Read the model definition and answer for the solid it produces. Units are mm, in the model's axes. Face numbers are marked on the shaded views. A direction names the side the tool comes from. Coordinates: 2 decimals unless noted, no trailing zeros. Loops run counter-clockwise (first coordinate to the right, second up) from the corner with the lowest first, then second, coordinate; pieces in that order, holes last. Notation, with made-up numbers: (-27.5, 36) -> (-8.5, 36) arc R26 ccw to (-8.5, 52) -> close; hole circle Ø4 at (6.25, -36). An arc over 180 degrees is marked (long way). Answer as a JSON object with one key per item and string values. Group by question number.
Q1. Straight lines are drawn through the part: line 1 along Y through (x, z) = (3.35, 68); line 2 along Y through (x, z) = (3.95, 68.5); line 3 along Z through (x, y) = (3.9, -13.5). For each, find the intervals that lie inside material, in ascending order. Write a range as [from, to].
Q2. The part is cut by section B-B on z = 68. Write down the section's boundary in (x, y) (3 decimals).
Q3. The part is cut by section A-A on y = 14.5. Write down the section's boundary in (x, z), and give its area (3 significant figures).
Q4. Determine the mould class of the marked faces 1, 2 and 3 for opening direction X: released by +X, released by -X, zero draft, split by the parting line, or undercut.
Q5. The part is cut by section D-D on x = 7.8. Write down the section's boundary in (y, z) (3 decimals).
Q6. For the marked faces 4, 5 and 6, determine the directions among +Z, -Z, +X, -X, +Y, -Y from which every point of the face is accessible in a straight line to the end or side of a thin tool.
Q7. Each of these flat-tipped pins is pushed along its axis until it touches: P1, Ø2.5, axis at x = 6.5, z = 68, coming from the +Y side (3 decimals); P2, Ø2.5, axis at y = 13.5, z = 68.5, coming from the +X side; P3, Ø4, axis at y = 14.5, z = 68, coming from the -X side; P4, Ø4, axis at y = -13.5, z = 69, coming from the +X side. Where does it stop, or does it pass through?
Q8. The part is cut by section C-C on x = 3.2. Write down the section's boundary in (y, z).
from build123d import *

# Parameters (mm, degrees)
PAD010_DEPTH            = 8
SKETCH006_R             = 1.5
POCKET013_DEPTH         = 5
FILLET007_R             = 2
BODY002_PITCH_ANGLE     = -90
BODY002_PLACEMENT_ANGLE = -180


with BuildPart() as part:
    # Sketch005 → Pad010 (new body)
    with BuildSketch(Plane.YZ):
        Polygon((-17, -5), (-11.875, -5), (-11.875, -1.6), (10.875, -1.6), (10.875, -5), (16, -5), (16, -7), (-17, -7), align=None)
    extrude(amount=PAD010_DEPTH)

    # Sketch006 (on Face7 of Pad010) → Pocket013 (cut)
    with BuildSketch(Plane.YX.offset(7)):
        with Locations((-14.5, 4)):
            Circle(SKETCH006_R)
        with Locations((13.5, 4)):
            Circle(SKETCH006_R)
    extrude(amount=-POCKET013_DEPTH, mode=Mode.SUBTRACT)

    # Fillet007
    fillet007_edges = [part.edges().sort_by_distance(p)[0] for p in [
        (8, -17, -6),
        (0, -17, -6),
        (8, 16, -6),
        (0, 16, -6),
    ]]
    fillet(fillet007_edges, radius=FILLET007_R)


with BuildPart() as part_1:
    # Body002 pitch: moved
    add(part.part.rotate(Axis((0, 0, 0), (0, 1, 0)), BODY002_PITCH_ANGLE))


with BuildPart() as part_2:
    # Body002 placement: moved
    add(part_1.part.moved(Location((9.75, 0, 64))).rotate(Axis((9.75, 0, 64), (0, 0, 1)), BODY002_PLACEMENT_ANGLE))


solid = part_2.part
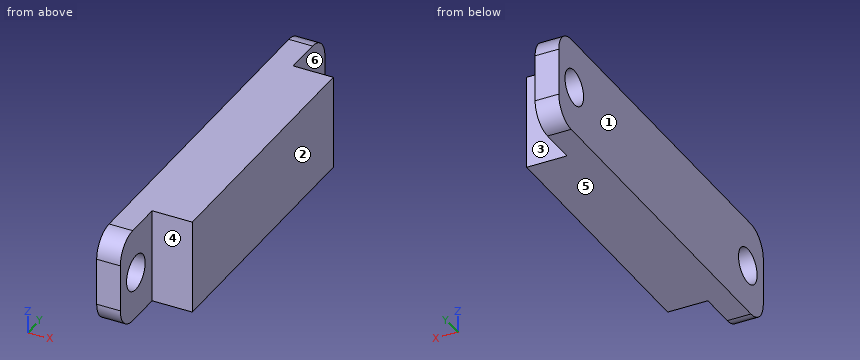
Final values:
{
 "1": {"line 1": "y = [-16, -15], [-12, 13], [16, 17]", "line 2": "y = [-16, -14.91], [-12.09, 13.09], [15.91, 17]", "line 3": "z = [64, 66.5], [69.5, 72]"},
 "2": {"outline": "(2.75, -16) -> (4.75, -16) -> (4.75, -15) -> (2.75, -15) -> close; (2.75, -12) -> (4.75, -12) -> (4.75, -10.875) -> (8.15, -10.875) -> (8.15, 11.875) -> (4.75, 11.875) -> (4.75, 13) -> (2.75, 13) -> close; (2.75, 16) -> (4.75, 16) -> (4.75, 17) -> (2.75, 17) -> close"},
 "3": {"outline": "(2.75, 64) -> (4.75, 64) -> (4.75, 66.5) -> (2.75, 66.5) -> close; (2.75, 69.5) -> (4.75, 69.5) -> (4.75, 72) -> (2.75, 72) -> close", "area": "10.0 mm2"},
 "4": {"face 1": "released by -X", "face 2": "released by +X", "face 3": "zero draft"},
 "5": {"outline": "(-10.875, 64) -> (11.875, 64) -> (11.875, 72) -> (-10.875, 72) -> close"},
 "6": {"face 4": "+Z, -Z, +X, -Y", "face 5": "-Z, +X, -X, +Y, -Y", "face 6": "+Z, -Z, +X, +Y"},
 "7": {"P1": "stops at y = 11.875", "P2": "stops at x = 4.75", "P3": "stops at x = 2.75", "P4": "stops at x = 4.75"},
 "8": {"outline": "(-16, 66) arc R2 ccw to (-14, 64) -> (15, 64) arc R2 ccw to (17, 66) -> (17, 70) arc R2 ccw to (15, 72) -> (-14, 72) arc R2 ccw to (-16, 70) -> close; hole circle Ø3 at (-13.5, 68); hole circle Ø3 at (14.5, 68)"}
}
